Verification items for this drawing (mm, ordinates from the low corner). Round coordinates to 2 decimals unless told otherwise and drop trailing zeros. Write each loop counter-clockwise with the first axis right and the second up, starting at its lowest first coordinate (ties: lowest second). Pieces come first, ordered by that corner, then holes. Notation, with made-up numbers: (5, 70.25) -> (12, 70.25) arc R19 ccw to (12, 102.25) -> close; hole circle Ø7 at (2, -18.5). An arc over 180 degrees is marked (long way). One line per item, written item: value.
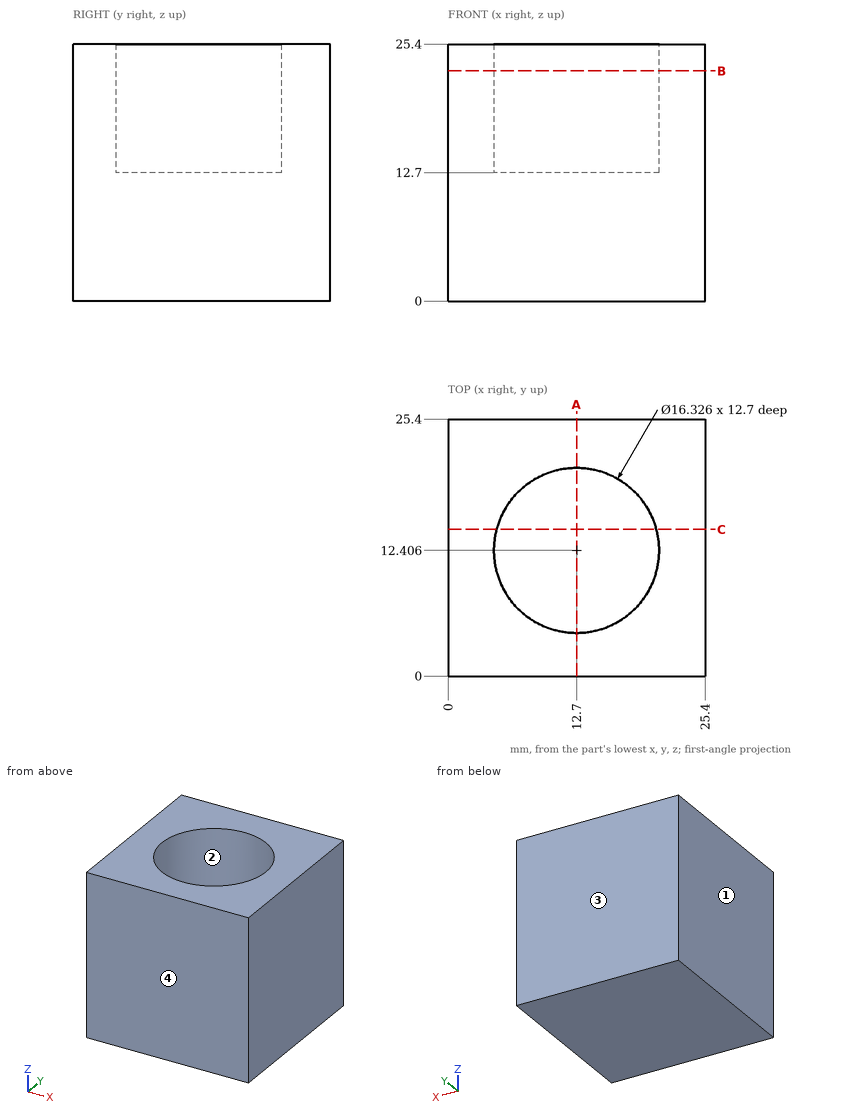
Item 1: Sectioned sample at B-B (z = 22.75). Enter the section's corners in (x, y), then the cut area to 3 significant figures.
Result set:
outline: (0, 0) -> (25.4, 0) -> (25.4, 25.4) -> (0, 25.4) -> close; hole circle Ø16.33 at (12.7, 12.41)
area: 436 mm^2
Item 2: Sectioned sample at A-A (x = 12.7). Enter the section's corners in (y, z).
Result set:
outline: (0, 0) -> (25.4, 0) -> (25.4, 25.4) -> (20.57, 25.4) -> (20.57, 12.7) -> (4.24, 12.7) -> (4.24, 25.4) -> (0, 25.4) -> close
Item 3: Material ranges on line 1 along Y through (x, z) = (12.7, 19.25); line 2 along Z through (x, y) = (6, 13); line 3 along X through (y, z) = (8.25, 18) (1 decimal), recorded low to high.
Result set:
line 1: 0 to 4.24, 20.57 to 25.4
line 2: 0 to 12.7
line 3: 0 to 5.7, 19.7 to 25.4
Item 4: Release check for a two-part mould opening along Y. For the marked faces 1, 2, 3 and 4 record: pulls with the +Y half, pulls with the -Y half, needs draft (parallel to the pull), parting line crosses it, or undercut.
Result set:
face 1: needs draft
face 2: undercut
face 3: pulls with the +Y half
face 4: pulls with the -Y half
Item 5: Depth check by flat-ended pin: pin 1 (1.5 mm diameter, centred on x = 9, y = 17.5, fed in from +Z). Enter the tip coordinate at first touch or a pass-through.
Result set:
pin 1: z = 12.7
Item 6: Sectioned sample at C-C (y = 14.5). Enter the section's corners in (x, z).
Result set:
outline: (0, 0) -> (25.4, 0) -> (25.4, 25.4) -> (20.59, 25.4) -> (20.59, 12.7) -> (4.81, 12.7) -> (4.81, 25.4) -> (0, 25.4) -> close
